Input: part model. Units: mm. Frame: model coordinates. A direction names the side the tool comes from. Round coordinates to 2 decimals unless told otherwise and drop trailing zeros. Order: outer loops, then holes, each group sorted by start corner. A loop starts at its lowest first (then second) coordinate and runs counter-clockwise, first axis right, second up. Notation, with made-up numbers: (32, 45) - (88, 45) arc R18 cw to (88, 74) - close; hole circle Ø2 at (73, 64.5). An arc over 180 degrees is marked (long way). One line per item, written item: value. Start each with the question number.
Autodesk Inventor part; units mm, degrees
ref_plane "YZ Plane" through (0, 0, 0) normal (1, 0, 0) x (0, 1, 0)
ref_plane "XZ Plane" through (0, 0, 0) normal (0, 1, 0) x (-1, 0, 0)
ref_plane "XY Plane" through (0, 0, 0) normal (0, 0, 1) x (1, 0, 0)
sketch "スケッチ1" plane through (0, 0, 0) normal (0, 0, 1) x (1, 0, 0)
  line L0 (-33.5, 13.5) -> (33.5, 13.5)
  line L1 (33.5, 13.5) -> (33.5, -13.5)
  line L2 (33.5, -13.5) -> (-33.5, -13.5)
  line L3 (-33.5, -13.5) -> (-33.5, 13.5)
  line L4 (-33.5, 13.5) -> (33.5, -13.5) construction
  line L5 (33.5, 13.5) -> (-33.5, -13.5) construction
  line L6 (-47, 0) -> (47.5, 0) construction
  line L7 (33.5, 4) -> (34, 4)
  line L8 (34, 4) -> (34, -4)
  line L9 (34, -4) -> (33.5, -4)
  line L10 (33.5, -4) -> (33.5, 4) construction
  line L11 (33.5, 4) -> (34, -4) construction
  line L12 (34, 4) -> (33.5, -4) construction
  line L13 (0, 18.9) -> (0, -18.9) construction
  line L14 (-20.5, 12.5) -> (20.5, 12.5)
  line L15 (20.5, 12.5) -> (20.5, 10)
  line L16 (20.5, 10) -> (-20.5, 10)
  line L17 (-20.5, 10) -> (-20.5, 12.5)
  line L18 (-20.5, 12.5) -> (20.5, 10) construction
  line L19 (20.5, 12.5) -> (-20.5, 10) construction
  line L20 (-20.5, -12.5) -> (20.5, -12.5)
  line L21 (20.5, -12.5) -> (20.5, -10)
  line L22 (20.5, -10) -> (-20.5, -10)
  line L23 (-20.5, -10) -> (-20.5, -12.5)
  line L24 (33.5, -4) -> (28.5, -4)
  line L25 (28.5, -4) -> (28.5, 4)
  line L26 (28.5, 4) -> (33.5, 4)
  point P0 (0, 0)
  point P1 (33.75, 0)
  point P2 (0, 11.25)
  dimension "d0" = 67
  dimension "d1" = 27
  dimension "d2" = 0.5
  dimension "d3" = 8
  dimension "d6" = 41
  dimension "d7" = 2.5
  dimension "d8" = 1
  dimension "d9" = 5
extrude "押し出し1" add sketch "スケッチ1" along normal blind 1.5 contours L0 L1 L26 L25 L24 L2 L3 | L1 L24 L25 L26 | L14 L15 L16 L17 | L23 L22 L21 L20
extrude "押し出し2" add sketch "スケッチ1" against normal blind 1.5 contours L7 L8 L9 L1 | L1 L24 L25 L26
extrude "押し出し3" add sketch "スケッチ1" against normal blind 12 contours L14 L15 L16 L17 | L23 L22 L21 L20
extrude "押し出し4" add sketch "スケッチ1" along normal blind 2 contours L14 L15 L16 L17 | L23 L22 L21 L20
properties part number "opencm9.04"
1. Set-up query: faces 5 (the face through (28.5, 0, -1)), 6 (the face through (0, 12.5, -6)), 7 (the face through (0, -12.5, -6)), 8 (the face through (0, 11, 2)), 9 (the face through (20.5, 11, -6)). Return all of +Z, -Z, +X, -X, +Y, -Y with unobstructed straight access to the full face (end or side cutting, diameter ignored); none if empty.
2. Section C-C (z = -11). Return the cut outline in (x, y).
3. Section D-D (y = 5.5). Return the cut outline in (x, z).
4. Section A-A (x = 19). Return the cut outline in (y, z).
5. Pull-direction query (Y, two-part tool) for faces 1 (the face through (0, 13.5, 1)), 2 (the face through (0, 10, -6)), 3 (the face through (0, -11, 2)), 4 (the face through (0, -10, -6)); classes: released by +Y, released by -Y, zero draft, split by the parting line, or undercut.
6. Pin query (flat end, axial travel): pin 1 (1.2 mm diameter, centred on y = -11.5, z = -5, fed in from +X); pin 2 (3 mm diameter, centred on y = 11.5, z = -4, fed in from -X); pin 3 (8 mm diameter, centred on x = -6, y = -5, fed in from +Z). Return the tip coordinate at first contact, or that it passes through.
7. Line query: line 1 (Y direction, x = 5, z = -10.5); line 2 (Z direction, x = 7, y = -8.5); line 3 (X direction, y = -11.5, z = -10.5). Output: solid intervals per line, ascending. Write a range as from..to.
8. Section B-B (y = -1.5). Return the cut outline in (x, z), then the cut area to 3 significant figures.
Solved:
1. face 5: -Z, -X, +Y, -Y
1. face 6: -Z, +X, -X, +Y
1. face 7: -Z, +X, -X, -Y
1. face 8: +Z, +X, -X, +Y, -Y
1. face 9: -Z, +X, +Y, -Y
2. outline: (-20.5, -12.5) - (20.5, -12.5) - (20.5, -10) - (-20.5, -10) - close; (-20.5, 10) - (20.5, 10) - (20.5, 12.5) - (-20.5, 12.5) - close
3. outline: (-33.5, 0) - (33.5, 0) - (33.5, 1.5) - (-33.5, 1.5) - close
4. outline: (-13.5, 0) - (-12.5, 0) - (-12.5, -12) - (-10, -12) - (-10, 0) - (10, 0) - (10, -12) - (12.5, -12) - (12.5, 0) - (13.5, 0) - (13.5, 1.5) - (12.5, 1.5) - (12.5, 2) - (10, 2) - (10, 1.5) - (-10, 1.5) - (-10, 2) - (-12.5, 2) - (-12.5, 1.5) - (-13.5, 1.5) - close
5. face 1: released by +Y
5. face 2: undercut
5. face 3: zero draft
5. face 4: undercut
6. pin 1: stops at x = 20.5
6. pin 2: stops at x = -20.5
6. pin 3: stops at z = 1.5
7. line 1: y = -12.5..-10, 10..12.5
7. line 2: z = 0..1.5
7. line 3: x = -20.5..20.5
8. outline: (-33.5, 0) - (28.5, 0) - (28.5, -1.5) - (34, -1.5) - (34, 0) - (33.5, 0) - (33.5, 1.5) - (-33.5, 1.5) - close
8. area: 109 mm²
